```python
from build123d import *

# Parameters (mm, degrees)
SKETCH1_R                   = 60
SKETCH1_R_2                 = 40
BOSS_EXTRUDE1_DEPTH         = 7
M3_CLEARANCE_HOLE1_D        = 3.4
BOSS_EXTRUDE3_START         = 5
SKETCH4_R                   = 60
SKETCH4_R_2                 = 50
BOSS_EXTRUDE3_DEPTH         = 5
BOSS_EXTRUDE4_START         = -12
BOSS_EXTRUDE4_DEPTH         = 12
TAP_DRILL_FOR_M4_TAP1_D     = 3.3
TAP_DRILL_FOR_M4_TAP1_DEPTH = 10
TAP_DRILL_FOR_M4_TAP1_TIP   = 0.991420021


with BuildPart() as part:
    # Sketch1 → Boss-Extrude1 (new body)
    with BuildSketch(Plane.XY):
        Circle(SKETCH1_R)
        Circle(SKETCH1_R_2, mode=Mode.SUBTRACT)
    extrude(amount=BOSS_EXTRUDE1_DEPTH)

    # M3 Clearance Hole1 (through all)
    with Locations(Plane.XY.offset(7)):
        with Locations((-31.466251763, 31.466251763), (0, 44.5), (31.466251763, 31.466251763), (44.5, 0), (31.466251763, -31.466251763), (0, -44.5), (-31.466251763, -31.466251763), (-44.5, 0)):
            Hole(M3_CLEARANCE_HOLE1_D / 2)

    # Sketch4 → Boss-Extrude3 (add)
    with BuildSketch(Plane(origin=(0, 0, 0), x_dir=(-1, 0, 0), z_dir=(0, 0, -1)).offset(BOSS_EXTRUDE3_START)):
        Circle(SKETCH4_R)
        Circle(SKETCH4_R_2, mode=Mode.SUBTRACT)
    extrude(amount=-BOSS_EXTRUDE3_DEPTH)

    # Sketch5 → Boss-Extrude4 (add)
    with BuildSketch(Plane.XY.offset(7).offset(BOSS_EXTRUDE4_START)):
        with BuildLine():
            Line((-60, 0), (-60, -62))
            Line((-60, -62), (60, -62))
            Line((60, -62), (60, 0))
            ThreePointArc((60, 0), (0, -60), (-60, 0))
        make_face()
    extrude(amount=BOSS_EXTRUDE4_DEPTH)

    # Tap Drill for M4 Tap1
    with Locations(Plane(origin=(0, -62, 0), x_dir=(-1, 0, 0), z_dir=(0, -1, 0))):
        with Locations((-50, -1), (0, -1), (25, -1), (50, -1), (-25, -1)):
            Hole(TAP_DRILL_FOR_M4_TAP1_D / 2, depth=TAP_DRILL_FOR_M4_TAP1_DEPTH)
            with Locations((0, 0, -(TAP_DRILL_FOR_M4_TAP1_DEPTH + TAP_DRILL_FOR_M4_TAP1_TIP / 2))):  # 118° drill point
                Cone(0, TAP_DRILL_FOR_M4_TAP1_D / 2, TAP_DRILL_FOR_M4_TAP1_TIP, mode=Mode.SUBTRACT)


solid = part.part
```
The model under review builds one solid part; all positions refer to its coordinate system, in mm. A direction names the side the tool comes from. Give positions to 0.01 mm unless a question says otherwise; leave off trailing zeros. Loops run counter-clockwise (first coordinate to the right, second up) from the corner with the lowest first, then second, coordinate; pieces in that order, holes last. Notation, with made-up numbers: (-2, 13.25) - (12, 13.25) arc R16 ccw to (12, 19.25) - close; hole circle Ø5 at (-7.75, 39). An arc over 180 degrees is marked (long way). Answer as a JSON object with one key per item and string values.
Q1. Add section B-B on x = 44.5. State the section outline as (y, z) points.
Worked out:
{"outline": "(-62, -5) - (-22.8, -5) - (-22.8, 0) - (-1.7, 0) - (-1.7, 7) - (-62, 7) - close; (1.7, 0) - (22.8, 0) - (22.8, -5) - (40.25, -5) - (40.25, 7) - (1.7, 7) - close"}
Q2. Mouldability with a two-part tool opening along X and no side actions: class faces 1 (the flat face through (-1, -62, 4)), 2 (the cylindrical face through (-8.67, -39.05, 3.45)), 3 (the cylindrical face through (-31.24, -29.78, 3.45)), 4 (the flat face through (60, -31, 1)) as +X half, -X half, draft (parallel to the pull), parting line (faces both ways), or undercut.
Worked out:
{"face 1": "draft", "face 2": "undercut", "face 3": "undercut", "face 4": "+X half"}
Q3. Add section A-A on y = -44.5. State the section outline as (x, z) points.
Worked out:
{"outline": "(-60, -5) - (-22.8, -5) - (-22.8, 0) - (-1.7, 0) - (-1.7, 7) - (-60, 7) - close; (1.7, 0) - (22.8, 0) - (22.8, -5) - (60, -5) - (60, 7) - (1.7, 7) - close"}
Q4. To check wall thickness, follow line 1 along Y through (x, z) = (0, 4); line 2 along Z through (x, y) = (0, -57); line 3 along Y through (x, z) = (-32.5, 2.5). State the ranges of each line that lie inside material, in increasing order.
Worked out:
{"line 1": "y = -62 to -46.2, -42.8 to -40, 40 to 42.8, 46.2 to 60", "line 2": "z = -5 to -0.65, 2.65 to 7", "line 3": "y = -62 to -32.82, -30.12 to -23.32, 23.32 to 30.12, 32.82 to 50.44"}
Q5. Insertion check: pin 1 (1.5 mm diameter, centred on y = 42.5, z = 0, fed in from -X); pin 2 (5.5 mm diameter, centred on x = 0, y = 44.5, fed in from -Z); pin 3 (5.5 mm diameter, centred on x = 0, z = 1, fed in from +Y). Each pin has a flat end and moves straight along its axis. Give the tip position at first contact, or say it passes through.
Worked out:
{"pin 1": "stops at x = -43.09", "pin 2": "stops at z = 0", "pin 3": "stops at y = 60"}
Q6. For faces 5 (the cylindrical face through (-47.69, 15.02, -2.54)), 6 (the cylindrical face through (23.35, -56.93, 0.93)), 7 (the cylindrical face through (0.37, -46.16, 3.45)), list the 3-axis set-ups (+Z, -Z, +X, -X, +Y, -Y) from which the entire face can be reached by the end or side of a thin tool; tool diameter is ignored.
Worked out:
{"face 5": "-Z", "face 6": "-Y", "face 7": "+Z, -Z"}
